Verification items for the finished model (mm, model axes). A direction names the side the tool comes from. Round coordinates to 2 decimals unless told otherwise and drop trailing zeros. Order: outer loops, then holes, each group sorted by start corner. A loop starts at its lowest first (then second) coordinate and runs counter-clockwise, first axis right, second up. Notation, with made-up numbers: M 14.25,24.25 L 51.25,24.25 A24 ccw 51.25,43.25 Z; hole C -1.75,80 d4. An arc over 180 degrees is marked long. Write item = value, one per line. Start each with the question number.
from build123d import *

# Parameters (mm, degrees)
BOSS_EXTRUDE1_DEPTH = 11.8
BOSS_EXTRUDE2_DEPTH = 4.5
SKETCH3_R           = 2.375
BOSS_EXTRUDE3_DEPTH = 3.4
CUT_EXTRUDE1_REACH  = 21.4
SKETCH4_R           = 1.25


with BuildPart() as part:
    # Sketch1 → Boss-Extrude1 (new body)
    with BuildSketch(Plane.XY):
        Polygon((0, 0), (22.5, 0), (22.5, 16.95), (27.4, 16.95), (27.4, 19.4), (22.5, 19.4), (22.5, 23.7), (0, 23.7), (0, 19.4), (-4.9, 19.4), (-4.9, 16.95), (0, 16.95), align=None)
    extrude(amount=BOSS_EXTRUDE1_DEPTH)

    # Sketch2 → Boss-Extrude2 (add)
    with BuildSketch(Plane(origin=(0, 23.7, 0), x_dir=(1, 0, 0), z_dir=(0, 1, 0))):
        with BuildLine():
            ThreePointArc((11.18220339, -3.271630287), (0, -5.9), (11.18220339, -8.528369713))
            ThreePointArc((11.18220339, -8.528369713), (14.5, -5.9), (11.18220339, -3.271630287))
        make_face()
    extrude(amount=BOSS_EXTRUDE2_DEPTH)

    # Sketch3 → Boss-Extrude3 (add)
    with BuildSketch(Plane(origin=(0, 28.2, 0), x_dir=(1, 0, 0), z_dir=(0, 1, 0))):
        with Locations((5.9, -5.9)):
            Circle(SKETCH3_R)
    extrude(amount=BOSS_EXTRUDE3_DEPTH)

    # Sketch4 → Cut-Extrude1 (cut, up to next)
    with BuildSketch(Plane(origin=(0, 19.4, 0), x_dir=(1, 0, 0), z_dir=(0, 1, 0)), mode=Mode.PRIVATE) as cut_extrude1_sk1:
        with Locations((-2.45, -5.9)):
            Circle(SKETCH4_R)
    cut_extrude1_tool1 = extrude(cut_extrude1_sk1.sketch, amount=-CUT_EXTRUDE1_REACH, mode=Mode.PRIVATE) & part.part
    add(cut_extrude1_tool1.solids().sort_by_distance((-2.45, 19.4, 5.9))[0], mode=Mode.SUBTRACT)
    # Sketch4 → Cut-Extrude1 (cut, up to next)
    with BuildSketch(Plane(origin=(0, 19.4, 0), x_dir=(1, 0, 0), z_dir=(0, 1, 0)), mode=Mode.PRIVATE) as cut_extrude1_sk2:
        with Locations((24.95, -5.9)):
            Circle(SKETCH4_R)
    cut_extrude1_tool2 = extrude(cut_extrude1_sk2.sketch, amount=-CUT_EXTRUDE1_REACH, mode=Mode.PRIVATE) & part.part
    add(cut_extrude1_tool2.solids().sort_by_distance((24.95, 19.4, 5.9))[0], mode=Mode.SUBTRACT)


solid = part.part
1) Scan lines: probe 1 along X at (y, z) = (18.95, 5.9); probe 2 along Z at (x, y) = (-2.45, 17.75); probe 3 along X at (y, z) = (8, 4). Record each from-to range of solid material in increasing order.
2) Cross-section at B-B, the plane z = 6.75. Enter the section's corners in (x, y).
3) Cross-section at D-D, the plane x = -3. Enter the section's corners in (y, z).
4) Access from +Z, -Z, +X, -X, +Y, -Y to the whole of each face (thin tool, end or side, straight path). Record for faces 1 (the cylindrical face through (0, 26, 6)), 2 (the flat face through (0, 9, 6)), 3 (the flat face through (1, 23.7, 1)), 4 (the flat face through (22.5, 8, 6)).
5) Gauge pin test, flat ends, axial feed: P1, Ø2, axis at y = 24.5, z = 9, coming from the -X side; P2, Ø6, axis at x = 12.5, z = 8, coming from the +Y side; P3, Ø3, axis at x = 24.95, z = 5.9, coming from the -Y side; P4, Ø2, axis at x = -2.45, z = 5.9, coming from the +Y side. Record the tip position at first contact, or that the pin passes through.
6) Cross-section at A-A, the plane x = 11.8. Enter the section's corners in (y, z).
7) Cross-section at C-C, the plane y = 18.5. Enter the section's corners in (x, z), then the cut area to 3 significant figures.
Geometry results:
q1.probe_1 = -4.9 to -3.7, -1.2 to 23.7, 26.2 to 27.4
q1.probe_2 = 0 to 4.65, 7.15 to 11.8
q1.probe_3 = 0 to 22.5
q2.outline = M -4.9,16.95 L -3.37,16.95 L -3.37,19.4 L -4.9,19.4 Z; M -1.53,16.95 L 0,16.95 L 0,0 L 22.5,0 L 22.5,16.95 L 24.03,16.95 L 24.03,19.4 L 22.5,19.4 L 22.5,23.7 L 14.36,23.7 L 14.36,28.2 L 8.12,28.2 L 8.12,31.6 L 3.68,31.6 L 3.68,28.2 L 0.06,28.2 L 0.06,23.7 L 0,23.7 L 0,19.4 L -1.53,19.4 Z; M 25.87,16.95 L 27.4,16.95 L 27.4,19.4 L 25.87,19.4 Z
q3.outline = M 16.95,0 L 19.4,0 L 19.4,4.78 L 16.95,4.78 Z; M 16.95,7.02 L 19.4,7.02 L 19.4,11.8 L 16.95,11.8 Z
q4.face_1 = +Y
q4.face_2 = +Z, -Z, -X, -Y
q4.face_3 = -Z, -X, +Y
q4.face_4 = +Z, -Z, +X, -Y
q5.P1 = 0
q5.P2 = 28.2
q5.P3 = 16.95
q5.P4 = through
q6.outline = M 0,0 L 23.7,0 L 23.7,3.2 L 28.2,3.2 L 28.2,8.6 L 23.7,8.6 L 23.7,11.8 L 0,11.8 Z
q7.outline = M -4.9,0 L 27.4,0 L 27.4,11.8 L -4.9,11.8 Z; hole C -2.45,5.9 d2.5; hole C 24.95,5.9 d2.5
q7.area = 371 mm^2
